from build123d import *

# Parameters (mm, degrees)
F1_DEPTH = 25.4
F2_DEPTH = 38.1
F3_DEPTH = 12.7
F5_DEPTH = 6.35


with BuildPart() as f1:
    # F0 (on Top) → F1 (new body)
    with BuildSketch(Plane.XY):
        with BuildLine():
            ThreePointArc((-50.8001835883, 0), (-55.449863437, 11.2253201513), (-66.6751835883, 15.875))
            Line((-66.6751835883, 15.875), (-66.6751835883, 9.525))
            ThreePointArc((-66.6751835883, 9.525), (-59.9399914975, 6.7351920908), (-57.1501835883, 0))
            ThreePointArc((-57.1501835883, 0), (-59.9399914975, -6.7351920908), (-66.6751835883, -9.525))
            Line((-66.6751835883, -9.525), (-66.6751835883, -15.875))
            ThreePointArc((-66.6751835883, -15.875), (-55.449863437, -11.2253201513), (-50.8001835883, 0))
        make_face()
        with BuildLine():
            Line((-66.6751835883, 9.525), (-66.6751835883, 15.875))
            ThreePointArc((-66.6751835883, 15.875), (-82.5501835883, 0), (-66.6751835883, -15.875))
            Line((-66.6751835883, -15.875), (-66.6751835883, -9.525))
            ThreePointArc((-66.6751835883, -9.525), (-76.2001835883, 0), (-66.6751835883, 9.525))
        make_face()
    extrude(amount=F1_DEPTH)



with BuildPart() as f2:
    # F0 (on Top) → F2 (new body)
    with BuildSketch(Plane.XY):
        with BuildLine():
            ThreePointArc((28.5748164117, -15.875), (12.6998164117, 0), (28.5748164117, 15.875))
            Line((28.5748164117, 15.875), (28.5748164117, 28.575))
            Line((28.5748164117, 28.575), (21.0879168484, 27.5767467249))
            ThreePointArc((21.0879168484, 27.5767467249), (-0.0001835883, 0), (21.0879168484, -27.5767467249))
            Line((21.0879168484, -27.5767467249), (28.5748164117, -28.575))
            Line((28.5748164117, -28.575), (28.5748164117, -15.875))
        make_face()
        with BuildLine():
            ThreePointArc((28.5748164117, 15.875), (39.800136563, 11.2253201513), (44.4498164117, 0))
            ThreePointArc((44.4498164117, 0), (39.800136563, -11.2253201513), (28.5748164117, -15.875))
            Line((28.5748164117, -15.875), (28.5748164117, -28.575))
            ThreePointArc((28.5748164117, -28.575), (48.7803926841, -20.2055762724), (57.1498164117, 0))
            ThreePointArc((57.1498164117, 0), (48.7803926841, 20.2055762724), (28.5748164117, 28.575))
            Line((28.5748164117, 28.575), (28.5748164117, 15.875))
        make_face()
    extrude(amount=F2_DEPTH)


with BuildPart() as f1_1:
    add(f1.part)

    add(f2.part)  # F3 merges F2
    # F0 (on Top) → F3 (join)
    with BuildSketch(Plane.XY):
        with BuildLine():
            ThreePointArc((21.0879168484, -27.5767467249), (-0.0001835883, 0), (21.0879168484, 27.5767467249))
            Line((21.0879168484, 27.5767467249), (-66.6751835883, 15.875))
            ThreePointArc((-66.6751835883, 15.875), (-55.449863437, 11.2253201513), (-50.8001835883, 0))
            ThreePointArc((-50.8001835883, 0), (-55.449863437, -11.2253201513), (-66.6751835883, -15.875))
            Line((-66.6751835883, -15.875), (21.0879168484, -27.5767467249))
        make_face()
    extrude(amount=F3_DEPTH)

    # F4 (on Front) → F5 (join, symmetric)
    with BuildSketch(Plane.XZ):
        Polygon((-50.8, 0), (0, 0), (4.6227602288, 0), (4.6227602288, 38.1), (0, 38.1), (-50.8, 25.4), (-54.4934645295, 25.4), (-54.4934645295, 0), align=None)
    extrude(amount=F5_DEPTH, both=True)


solid = f1_1.part
CAD build for the part. Positions are in the model's coordinates, mm. A direction names the side the tool comes from. Give positions to 0.01 mm unless a question says otherwise; leave off trailing zeros. Loops run counter-clockwise (first coordinate to the right, second up) from the corner with the lowest first, then second, coordinate; pieces in that order, holes last. Notation, with made-up numbers: M 18.5,-3 L 68.5,-3 A34 cw 68.5,29 Z; hole C 30,16 d9. An arc over 180 degrees is marked long. Write each question's results on one line, items separated by ' | '.
Q1. Mould opens along X. For faces 6 (the face through (-26, 6.35, 23)), 7 (the face through (-9.134, -23.547, 10.317)), 8 (the face through (-14, 0, 0)) say: pulls with the +X half, pulls with the -X half, needs draft (parallel to the pull), parting line crosses it, or undercut.
Geometry check:
face 6: undercut | face 7: pulls with the -X half | face 8: needs draft
Q2. Which spindle directions (+Z, -Z, +X, -X, +Y, -Y) get a long thin tool onto all of the face, cutting with end or side? Do faces 1 (the face through (-23, -14, 12.7)), 2 (the face through (-57.59, -2.86, 12.52)), 3 (the face through (-67, -10, 25.4)), 4 (the face through (-23, 15, 12.7)), 5 (the face through (-7.8, 23.725, 10.317)). Say none if no direction does.
Geometry check:
face 1: +Z, -Y | face 2: +Z, -Z | face 3: +Z, -X, +Y, -Y | face 4: +Z, +Y | face 5: +Z, -Z, -X, +Y
Q3. Band-saw the part on C-C on y = 12.5. Write the cut outline in (x, z).
Geometry check:
outline: M -76.46,0 L 18.79,0 L 18.79,38.1 L 2.88,38.1 L 2.88,12.7 L -56.89,12.7 L -56.89,25.4 L -76.46,25.4 Z; M 38.36,0 L 54.27,0 L 54.27,38.1 L 38.36,38.1 Z
Q4. Band-saw the part on A-A on z = 36.5. Write the cut outline in (x, y) (3 decimals).
Geometry check:
outline: M -6.4,-6.35 L 0.714,-6.35 A28.575 ccw 21.088,-27.577 L 28.575,-28.575 A28.575 ccw 28.575,28.575 L 21.088,27.577 A28.575 ccw 0.714,6.35 L -6.4,6.35 Z; hole C 28.575,0 d31.75
Q5. Band-saw the part on D-D on x = 6.5. Write the cut outline in (y, z).
Geometry check:
outline: M -25.63,0 L 25.63,0 L 25.63,12.7 L 18.14,12.7 L 18.14,38.1 L -18.14,38.1 L -18.14,12.7 L -25.63,12.7 Z
Q6. Flat gauge pins, fed straight in: P1, Ø6.5, axis at x = -16, y = -19, coming from the +Z side; P2, Ø20.5, axis at x = -23, z = 29, coming from the -Y side; P3, Ø5, axis at y = -17.5, z = 14.5, coming from the +X side. Where does each tip first touch, or does it go through?
Geometry check:
P1: stops at z = 12.7 | P2: stops at y = -6.35 | P3: stops at x = 52.9
Q7. Band-saw the part on B-B on z = 5. Write the cut outline in (x, y) (3 decimals).
Geometry check:
outline: M -66.675,-15.875 L 28.575,-28.575 A28.575 ccw 28.575,28.575 L -66.675,15.875 A15.875 ccw Z; hole C -66.675,0 d19.05; hole C 28.575,0 d31.75
Q8. Probe probe 1 along Y at (x, z) = (29.5, 36); probe 2 along X at (y, z) = (-3.5, 11.5); probe 3 along Y at (x, z) = (-50.5, 23). List the from-to ranges inside material, lowest first.
Geometry check:
probe 1: y = -28.56 to -15.85, 15.85 to 28.56 | probe 2: x = -82.16 to -75.53, -57.82 to 13.09, 44.06 to 56.93 | probe 3: y = -6.35 to 6.35
